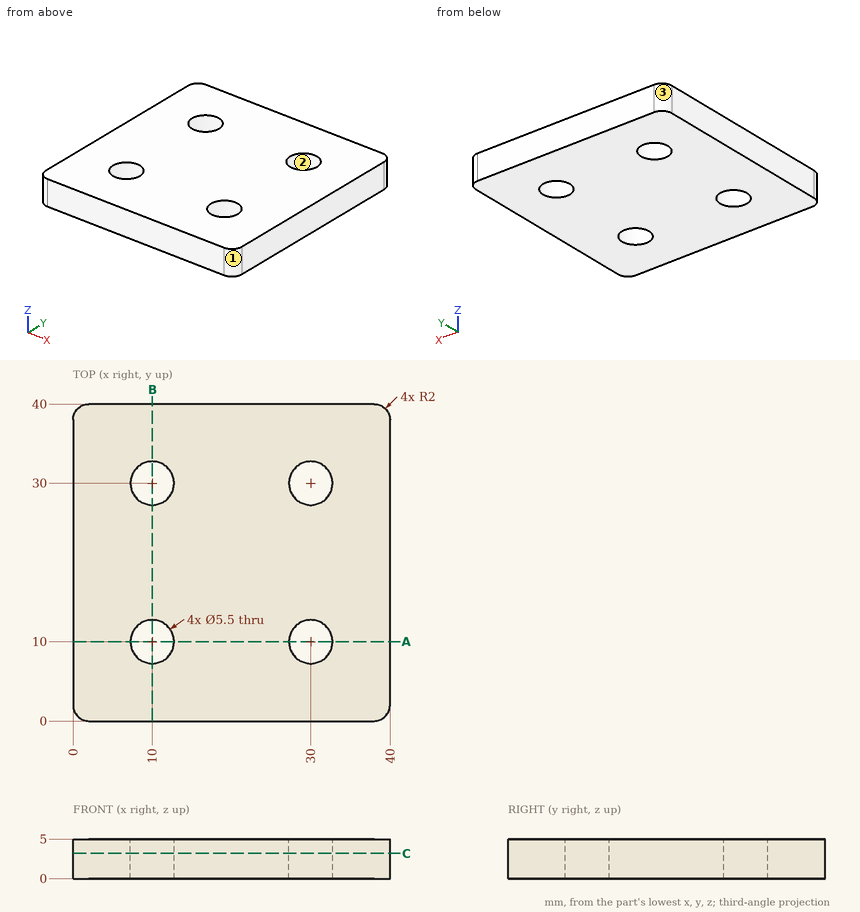
For this review, use the dimensioned drawing (mm, ordinates from the lowest corner) and the shaded views. Give positions to 0.01 mm unless a question says otherwise; leave off trailing zeros. Order: outer loops, then holes, each group sorted by start corner. A loop starts at its lowest first (then second) coordinate and runs counter-clockwise, first axis right, second up. Notation, with made-up numbers: (29, 25.25) - (76, 25.25) arc R13 ccw to (76, 44.25) - close; hole circle Ø10 at (48, 30). An arc over 180 degrees is marked (long way). Use a Markdown table: item, result. Add a question column.
(1) Wall thickness on probe 1 along X at (y, z) = (10, 3.5); probe 2 along X at (y, z) = (11, 3.05): over which ranges is each line inside the solid? List them lowest first. Write a range as [from, to].
(2) Mouldability with a two-part tool opening along X and no side actions: class the marked faces 1, 2 and 3 as +X half, -X half, draft (parallel to the pull), parting line (faces both ways), or undercut.
(3) Add section A-A on y = 10. Give the boundary of the cut face in (x, z).
(4) Add section C-C on z = 3.2. Give the boundary of the cut face in (x, y), then the cut area to 3 significant figures.
(5) Clearance check with a flat-ended pin moving along its axis: P1, Ø5, axis at x = 30, y = 10, coming from the +Z side. State where the tip first meets the part, or that it passes through.
Report:
| question | item | result |
|---|---|---|
| 1 | probe 1 | x = [0, 7.25], [12.75, 27.25], [32.75, 40] |
| 1 | probe 2 | x = [0, 7.44], [12.56, 27.44], [32.56, 40] |
| 2 | face 1 | +X half |
| 2 | face 2 | undercut |
| 2 | face 3 | -X half |
| 3 | outline | (0, 0) - (7.25, 0) - (7.25, 5) - (0, 5) - close; (12.75, 0) - (27.25, 0) - (27.25, 5) - (12.75, 5) - close; (32.75, 0) - (40, 0) - (40, 5) - (32.75, 5) - close |
| 4 | outline | (0, 2) arc R2 ccw to (2, 0) - (38, 0) arc R2 ccw to (40, 2) - (40, 38) arc R2 ccw to (38, 40) - (2, 40) arc R2 ccw to (0, 38) - close; hole circle Ø5.5 at (10, 10); hole circle Ø5.5 at (10, 30); hole circle Ø5.5 at (30, 10); hole circle Ø5.5 at (30, 30) |
| 4 | area | 1,500 mm² |
| 5 | P1 | passes through |
